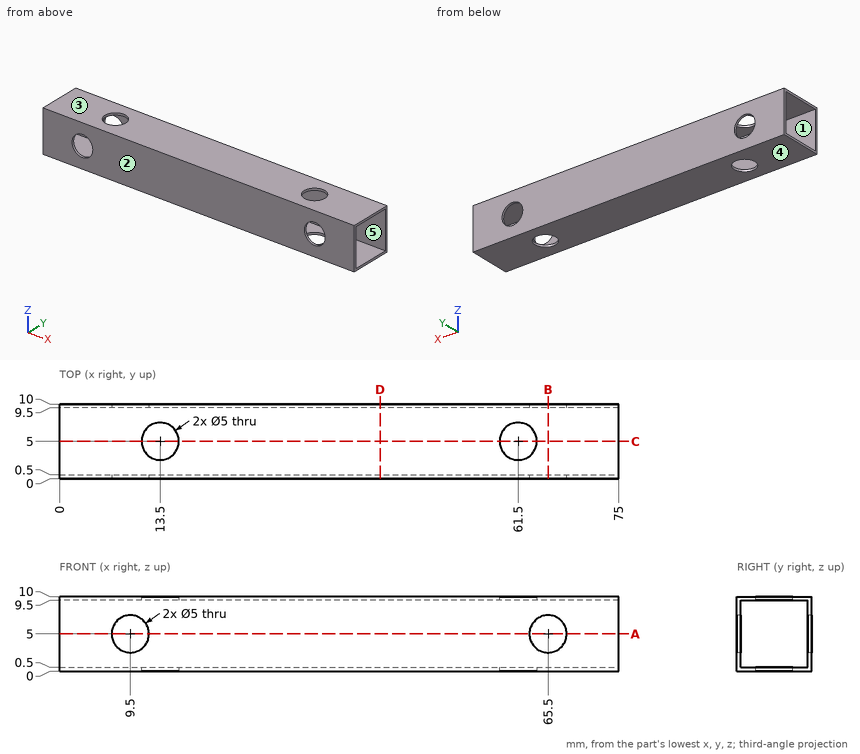
Answer from the drawing. Dimensions are ordinates in mm from the lowest x, y and z of the part. A direction names the side the tool comes from. Round coordinates to 2 decimals unless told otherwise and drop trailing zeros. Loops run counter-clockwise (first coordinate to the right, second up) from the corner with the lowest first, then second, coordinate; pieces in that order, holes last. Notation, with made-up numbers: M 14.5,39 L 21.5,39 A20 cw 21.5,51 Z; hole C 89,59 d4. An arc over 180 degrees is marked long. One line per question, with ' | ' between items. Start each with the question number.
(1) For a pull along Z with two mould halves and no side action, classify the marked faces 3, 4 and 5 as released by +Z, released by -Z, zero draft, split by the parting line, or undercut.
(2) A cutting plane is placed at C-C on y = 5. Write down the section's boundary in (x, z).
(3) A cutting plane is placed at B-B on x = 65.5. Write down the section's boundary in (y, z).
(4) A cutting plane is placed at D-D on x = 43. Write down the section's boundary in (y, z), plus the area to 3 significant figures.
(5) Find the intervals of material crossed by line 1 (Z direction, x = 64, y = 6.5); line 2 (Z direction, x = 9.5, y = 9.7), in increasing order.
(6) A cutting plane is placed at A-A on z = 5. Write down the section's boundary in (x, y).
(7) A tool of negligible diameter and unlimited length cuts with its end or side. For the marked faces 1 and 2, from which of +Z, -Z, +X, -X, +Y, -Y can it reach the whole face along a straight path? Write none if from no direction.
Geometry check:
1) face 3: released by +Z | face 4: released by -Z | face 5: undercut
2) outline: M 0,0 L 11,0 L 11,0.5 L 0,0.5 Z; M 0,9.5 L 11,9.5 L 11,10 L 0,10 Z; M 16,0 L 59,0 L 59,0.5 L 16,0.5 Z; M 16,9.5 L 59,9.5 L 59,10 L 16,10 Z; M 64,0 L 75,0 L 75,0.5 L 64,0.5 Z; M 64,9.5 L 75,9.5 L 75,10 L 64,10 Z
3) outline: M 0,0 L 10,0 L 10,2.5 L 9.5,2.5 L 9.5,0.5 L 0.5,0.5 L 0.5,2.5 L 0,2.5 Z; M 0,7.5 L 0.5,7.5 L 0.5,9.5 L 9.5,9.5 L 9.5,7.5 L 10,7.5 L 10,10 L 0,10 Z
4) outline: M 0,0 L 10,0 L 10,10 L 0,10 Z; hole M 0.5,0.5 L 9.5,0.5 L 9.5,9.5 L 0.5,9.5 Z | area: 19.0 mm²
5) line 1: z = 0 to 0.5, 9.5 to 10 | line 2: z = 0 to 2.5, 7.5 to 10
6) outline: M 0,0 L 7,0 L 7,0.5 L 0,0.5 Z; M 0,9.5 L 7,9.5 L 7,10 L 0,10 Z; M 12,0 L 63,0 L 63,0.5 L 12,0.5 Z; M 12,9.5 L 63,9.5 L 63,10 L 12,10 Z; M 68,0 L 75,0 L 75,0.5 L 68,0.5 Z; M 68,9.5 L 75,9.5 L 75,10 L 68,10 Z
7) face 1: +X, -X | face 2: +Z, -Z, +X, -X, -Y
